Autodesk Inventor part; units mm, degrees
ref_plane "YZ Plane" through (0, 0, 0) normal (1, 0, 0) x (0, 1, 0)
ref_plane "XZ Plane" through (0, 0, 0) normal (0, 1, 0) x (-1, 0, 0)
ref_plane "XY Plane" through (0, 0, 0) normal (0, 0, 1) x (1, 0, 0)
sketch "Sketch1" plane through (0, 0, 0) normal (0, 0, 1) x (1, 0, 0)
  arc A0 (11.7049, -23.2932) -> (16.7049, -28.2932) centre (16.7049, -23.2932) ccw
  line L0 (16.7049, -28.2932) -> (23.1049, -28.2932)
  line L1 (23.1049, -28.2932) -> (23.1049, -19.2932)
  line L2 (23.1049, -19.2932) -> (29.5049, -19.2932)
  line L3 (29.5049, -19.2932) -> (29.5049, -28.2932)
  line L4 (29.5049, -28.2932) -> (35.5049, -28.2932)
  line L5 (35.5049, -28.2932) -> (35.5049, -13.2932)
  line L6 (35.5049, -13.2932) -> (23.1049, -13.2932)
  line L7 (23.1049, -13.2932) -> (23.1049, 2.1068)
  line L8 (23.1049, 2.1068) -> (29.5049, 2.1068)
  line L9 (29.5049, 2.1068) -> (29.5049, -6.8932)
  line L10 (29.5049, -6.8932) -> (35.5049, -6.8932)
  line L11 (35.5049, -6.8932) -> (35.5049, 8.1068)
  line L12 (35.5049, 8.1068) -> (18.5049, 8.1068)
  line L13 (18.5049, 8.1068) -> (18.5049, 3.1068)
  line L14 (18.5049, 3.1068) -> (12.1049, 3.1068)
  line L15 (12.1049, 3.1068) -> (12.1049, 8.1068)
  line L16 (12.1049, 8.1068) -> (-11.8951, 8.1068)
  line L17 (-11.8951, 8.1068) -> (-11.8951, 3.1068)
  line L18 (-11.8951, 3.1068) -> (-18.2951, 3.1068)
  line L19 (-18.2951, 3.1068) -> (-18.2951, 8.1068)
  line L20 (-18.2951, 8.1068) -> (-42.2951, 8.1068)
  line L21 (-42.2951, 8.1068) -> (-42.2951, 3.1068)
  line L22 (-42.2951, 3.1068) -> (-48.6951, 3.1068)
  line L23 (-48.6951, 3.1068) -> (-48.6951, 8.1068)
  line L24 (-48.6951, 8.1068) -> (-72.4951, 8.1068)
  line L25 (-72.4951, 8.1068) -> (-72.4951, 3.1068)
  line L26 (-72.4951, 3.1068) -> (-78.8951, 3.1068)
  line L27 (-78.8951, 3.1068) -> (-78.8951, 8.1068)
  line L28 (-78.8951, 8.1068) -> (-81.8951, 8.1068)
  line L29 (-81.8951, 8.1068) -> (-81.8951, 17.1068)
  arc A1 (-81.8951, 17.1068) -> (-87.8951, 17.1068) centre (-84.8951, 17.1068) ccw
  line L30 (-87.8951, 17.1068) -> (-87.8951, -11.8932)
  line L31 (-87.8951, -11.8932) -> (6.7049, -11.8932)
  arc A2 (11.7049, -16.8932) -> (6.7049, -11.8932) centre (6.7049, -16.8932) ccw
  line L32 (11.7049, -16.8932) -> (11.7049, -23.2932)
  circle A3 centre (-45.4951, -4.3932) radius 1.5
  circle A4 centre (15.3049, -4.3932) radius 1.5
  point P0 (0, 0)
extrude "Extrusion1" add sketch "Sketch1" along normal blind 6
properties part number "spoolHolder_a"
Model file for the job. Use its own axes, mm. A direction names the side the tool comes from. Coordinates: 2 decimals unless noted, no trailing zeros. Order: outer loops, then holes, each group sorted by start corner. A loop starts at its lowest first (then second) coordinate and runs counter-clockwise, first axis right, second up. Notation, with made-up numbers: (46, -39.75) -> (76, -39.75) arc R18 ccw to (76, -34.75) -> close; hole circle Ø4 at (89, -33.75). An arc over 180 degrees is marked (long way). Answer as a JSON object with one key per item and string values. Group by question number.
1) Pull direction X, two halves, no side cores. Call faces 4 (the face through (13.21, -26.87, 2.96)), 5 (the face through (-42.295, 6, 3)), 6 (the face through (29, -13.293, 3)): +X half, -X half, draft (parallel to the pull), parting line (faces both ways), or undercut.
2) Which spindle directions (+Z, -Z, +X, -X, +Y, -Y) get a long thin tool onto all of the face, cutting with end or side? Do faces 1 (the face through (-18.295, 6, 3)), 2 (the face through (27, 8.107, 3)), 3 (the face through (26, -19.293, 3)). Say none if no direction does.
3) Drill centre lines: L1, parallel to X at y = 1, z = 0.75; L2, parallel to X at y = 3.5, z = 3; L3, parallel to X at y = -20, z = 2.85. Where is each one in solid material? Low to high.
4) Cut at C-C, the plane z = 3.1. Count the separate pieces of the cut face and the enclosed holes in it, then the cut area to 3 significant figures.
5) Flat gauge pins, fed straight in: pin 1 (2.5 mm diameter, centred on x = -80, z = 4.5, fed in from +Y); pin 2 (3.5 mm diameter, centred on x = 15.3, y = -4.39, fed in from -Z); pin 3 (3 mm diameter, centred on y = 11, z = 1.5, fed in from +X); pin 4 (3 mm diameter, centred on x = -53, z = 3.5, fed in from -Y). Where does each tip first touch, or does it go through?
6) Cut at B-B, the plane y = 10.5. Write the cut outline in (x, z).
7) Cut at A-A, the plane x = -75. Write the cut outline in (y, z).
Check values:
{
 "1": {"face 4": "-X half", "face 5": "undercut", "face 6": "draft"},
 "2": {"face 1": "+Z, -Z, +Y", "face 2": "+Z, -Z, +X, +Y", "face 3": "+Z, -Z, -Y"},
 "3": {"L1": "x = -87.9 to 23.1, 29.5 to 35.5", "L2": "x = -87.9 to -78.9, -72.5 to -48.7, -42.3 to -18.3, -11.9 to 12.1, 18.5 to 35.5", "L3": "x = 11.7 to 23.1, 29.5 to 35.5"},
 "4": {"separate pieces": "1", "enclosed holes": "2", "area": "2,590 mm²"},
 "5": {"pin 1": "stops at y = 8.11", "pin 2": "stops at z = 0", "pin 3": "stops at x = -81.9", "pin 4": "stops at y = -11.89"},
 "6": {"outline": "(-87.9, 0) -> (-81.9, 0) -> (-81.9, 6) -> (-87.9, 6) -> close"},
 "7": {"outline": "(-11.89, 0) -> (3.11, 0) -> (3.11, 6) -> (-11.89, 6) -> close"}
}
